Verification items for this drawing (mm, ordinates from the low corner). A direction names the side the tool comes from. Round coordinates to 2 decimals unless told otherwise and drop trailing zeros. Write each loop counter-clockwise with the first axis right and the second up, starting at its lowest first coordinate (ties: lowest second). Pieces come first, ordered by that corner, then holes. Notation, with made-up numbers: (36.5, -18) -> (47.5, -18) arc R18 cw to (47.5, 2) -> close; hole circle Ø5 at (54, 42). An arc over 180 degrees is marked (long way). Return JSON: item names as keys, results as strings. Group by question number.
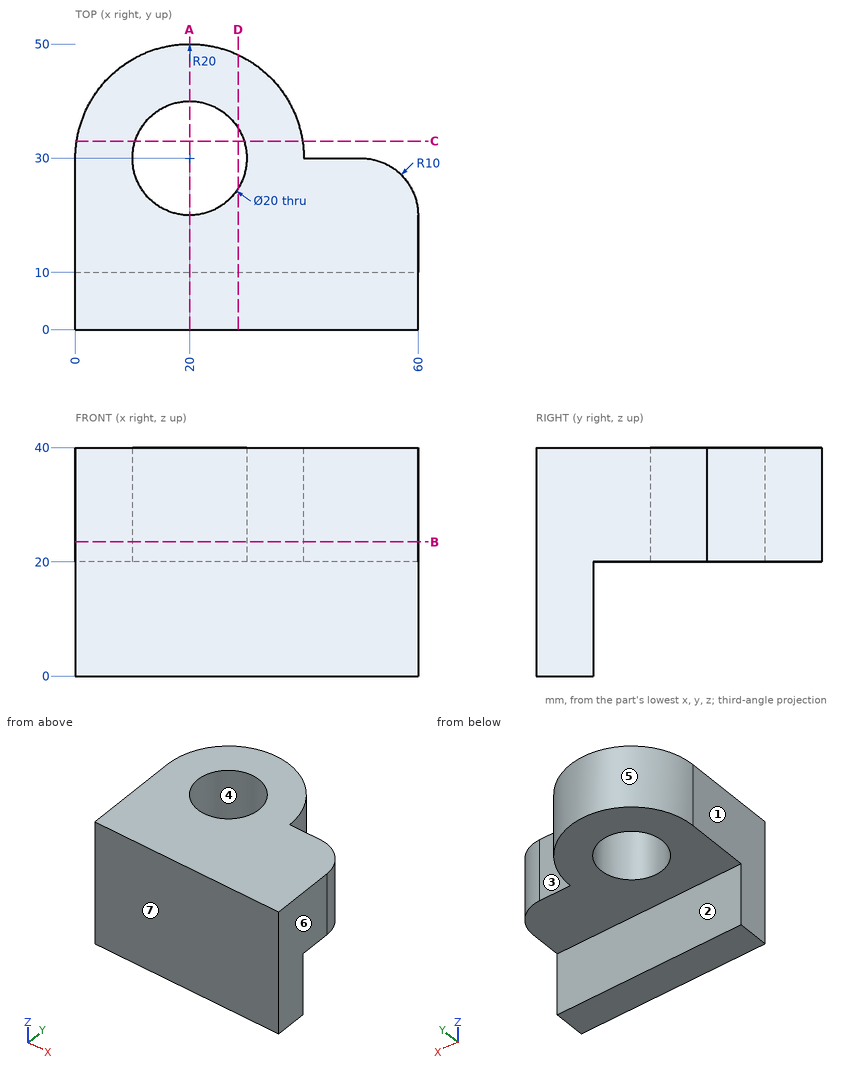
1) Tool access check on the marked faces 1, 2 and 3. Record the directions out of +Z, -Z, +X, -X, +Y, -Y that give a thin tool (end or side, any length) a straight path to the whole face; none if there is none.
2) Mould release check, pull along Y, two halves, no side actions. Record for the marked faces 4, 5, 6 and 7: +Y half, -Y half, draft (parallel to the pull), parting line (faces both ways), or undercut.
3) Sectioned sample at B-B on z = 23.5. Enter the section's corners in (x, y), and give its area (3 significant figures).
4) Sectioned sample at A-A on x = 20. Enter the section's corners in (y, z), and give its area (3 significant figures).
5) Sectioned sample at C-C on y = 33. Enter the section's corners in (x, z).
6) Material ranges on probe 1 along Y at (x, z) = (20, 28); probe 2 along Z at (x, y) = (5, 37); probe 3 along Y at (x, z) = (52.5, 17.5), recorded low to high. Write a range as [from, to].
7) Sectioned sample at D-D on x = 28.5. Enter the section's corners in (y, z).
8) Go/stop test with flat-tipped pins: P1, Ø23, axis at x = 20, y = 30, coming from the -Z side; P2, Ø12, axis at x = 42.5, z = 22.5, coming from the +Y side; P3, Ø3, axis at x = 43.5, z = 27.5, coming from the +Y side. Record where each tip stops, or that it passes through.
Evaluation:
{
 "1": {"face 1": "+Z, -Z, -X, +Y, -Y", "face 2": "-Z, +X, -X, +Y", "face 3": "+Z, -Z, +X, +Y"},
 "2": {"face 4": "undercut", "face 5": "+Y half", "face 6": "draft", "face 7": "-Y half"},
 "3": {"outline": "(0, 0) -> (60, 0) -> (60, 20) arc R10 ccw to (50, 30) -> (40, 30) arc R20 ccw to (0, 30) -> close; hole circle Ø20 at (20, 30)", "area": "2,090 mm2"},
 "4": {"outline": "(0, 0) -> (10, 0) -> (10, 20) -> (20, 20) -> (20, 40) -> (0, 40) -> close; (40, 20) -> (50, 20) -> (50, 40) -> (40, 40) -> close", "area": "800 mm2"},
 "5": {"outline": "(0.23, 20) -> (10.46, 20) -> (10.46, 40) -> (0.23, 40) -> close; (29.54, 20) -> (39.77, 20) -> (39.77, 40) -> (29.54, 40) -> close"},
 "6": {"probe 1": "y = [0, 20], [40, 50]", "probe 2": "z = [20, 40]", "probe 3": "y = [0, 10]"},
 "7": {"outline": "(0, 0) -> (10, 0) -> (10, 20) -> (24.73, 20) -> (24.73, 40) -> (0, 40) -> close; (35.27, 20) -> (48.1, 20) -> (48.1, 40) -> (35.27, 40) -> close"},
 "8": {"P1": "stops at z = 20", "P2": "stops at y = 41.3", "P3": "stops at y = 30"}
}
